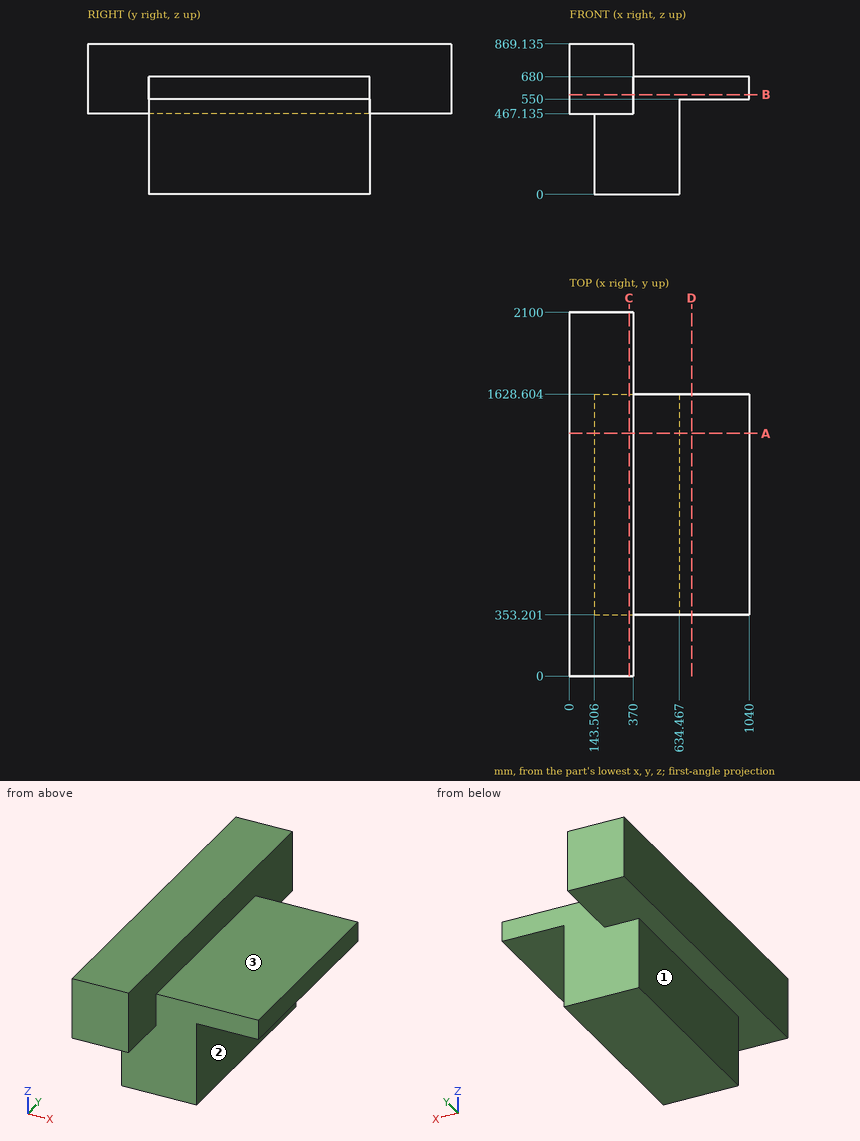
Could you check a few things on this drawing? It's one solid part, dimensions in mm from its lowest x, y, z. A direction names the side the tool comes from. Give positions to 0.01 mm unless a question says otherwise; leave off trailing zeros. Write each loop counter-clockwise with the first axis right and the second up, starting at its lowest first coordinate (ties: lowest second). Pieces come first, ordered by that corner, then holes. Notation, with made-up numbers: (-16, -14) -> (-7, -14) arc R7 ccw to (-7, -4) -> close; hole circle Ø6 at (38.25, 66.25). An arc over 180 degrees is marked (long way). Write each question's results on one line, items separated by ' | '.
1. I want a section at A-A, the plane y = 1402. Write out the boundary of the cut face in (x, z) (1 decimal).
Check sheet entries:
outline: (0, 467.1) -> (143.5, 467.1) -> (143.5, 0) -> (634.5, 0) -> (634.5, 550) -> (1040, 550) -> (1040, 680) -> (370, 680) -> (370, 869.1) -> (0, 869.1) -> close
2. On a 3-axis mill with a long thin cutter (end or side, diameter ignored), from which of +Z, -Z, +X, -X, +Y, -Y can I reach the whole of each face in a straight line? I mean the marked faces 1, 2 and 3. Say none if no direction works.
Check sheet entries:
face 1: -Z, -X, +Y, -Y | face 2: -Z, +X, +Y, -Y | face 3: +Z, +X, +Y, -Y
3. I want a section at B-B, the plane z = 577. Write out the boundary of the cut face in (x, y) (1 decimal), then the cut area to 3 significant figures.
Check sheet entries:
outline: (0, 0) -> (370, 0) -> (370, 353.2) -> (1040, 353.2) -> (1040, 1628.6) -> (370, 1628.6) -> (370, 2100) -> (0, 2100) -> close | area: 1,630,000 mm²
4. I want a section at D-D, the plane x = 706.5. Write out the boundary of the cut face in (y, z) (1 decimal).
Check sheet entries:
outline: (353.2, 550) -> (1628.6, 550) -> (1628.6, 680) -> (353.2, 680) -> close
5. I need wall thicknesses on L1, parallel to X at y = 1586.5, z = 351.5 (1 decimal); L2, parallel to Z at x = 575, y = 787; L3, parallel to Y at x = 209.5, z = 117 (1 decimal). Which ranges of each line are inside material? Lowest first, please.
Check sheet entries:
L1: x = 143.5 to 634.5 | L2: z = 0 to 680 | L3: y = 353.2 to 1628.6
6. Will these pins go through, and if not, where does the flat tip stop? pin 1 Ø4 at (y, z) = (965, 412.5) entering from -X; pin 2 Ø1.5 at (x, y) = (807.5, 1552) entering from -Z; pin 3 Ø12 at (x, z) = (192.5, 190.5) entering from -Y.
Check sheet entries:
pin 1: stops at x = 143.51 | pin 2: stops at z = 550 | pin 3: stops at y = 353.2
7. I want a section at C-C, the plane x = 345.5. Write out the boundary of the cut face in (y, z) (1 decimal).
Check sheet entries:
outline: (0, 467.1) -> (353.2, 467.1) -> (353.2, 0) -> (1628.6, 0) -> (1628.6, 467.1) -> (2100, 467.1) -> (2100, 869.1) -> (0, 869.1) -> close
